Design review of the part built by this model. Coordinates are the model's own, in mm. Face numbers are marked on the shaded views. A direction names the side the tool comes from. Coordinates: 2 decimals unless noted, no trailing zeros. Loops run counter-clockwise (first coordinate to the right, second up) from the corner with the lowest first, then second, coordinate; pieces in that order, holes last. Notation, with made-up numbers: M 2,-10.75 L 13,-10.75 A22 ccw 13,26.25 Z; hole C 21.25,84.25 d11. An arc over 180 degrees is marked long. One line per item, written item: value.
```python
from build123d import *

# Parameters (mm, degrees)
SKETCH1_R                = 1.6
BOSS_EXTRUDE1_DEPTH      = 10
CUT_EXTRUDE1_DEPTH       = 51.495476
FILLET1_R                = 0.5
BOSS_EXTRUDE2_DEPTH      = 10
BOSS_EXTRUDE2_DEPTH_BACK = 20
SKETCH3_R                = 1.5
SKETCH4_W                = 10
SKETCH4_H                = 10
CUT_EXTRUDE3_DEPTH       = 54.383453
SKETCH5_W                = 8.66368
SKETCH5_H                = 10
CUT_EXTRUDE5_DEPTH       = 54.831153
FILLET3_R                = 0.5
FILLET4_R                = 1


with BuildPart() as part:
    # Sketch1 → Boss-Extrude1 (new body)
    with BuildSketch(Plane(origin=(0, 0, 0), x_dir=(1, 0, 0), z_dir=(0, 1, 0))):
        with BuildLine():
            Line((0, 0), (23.162951, -23.162951))
            ThreePointArc((23.162951, -23.162951), (23.813269, -26.432322), (21.041631, -28.284271))
            Line((21.041631, -28.284271), (0, -28.284271))
            Line((0, -28.284271), (0, -34.284271))
            Line((0, -34.284271), (30.698485, -34.284271))
            ThreePointArc((30.698485, -34.284271), (35.317882, -31.197688), (34.234019, -25.748737))
            Line((34.234019, -25.748737), (4.242641, 4.242641))
            Line((4.242641, 4.242641), (0, 0))
        make_face()
        with Locations(Location((31.905592, -29.784271, 0), (0, 0, 270))):
            Circle(SKETCH1_R, mode=Mode.SUBTRACT)
    extrude(amount=BOSS_EXTRUDE1_DEPTH)

    # Sketch2 → Cut-Extrude1 (cut, through all)
    with BuildSketch(Plane(origin=(0, 10, 0), x_dir=(1, 0, 0), z_dir=(0, 1, 0))):
        with BuildLine():
            Line((1.414214, -1.414214), (9.899495, -9.899495))
            ThreePointArc((9.899495, -9.899495), (7.071068, -4.242641), (1.414214, -1.414214))
        make_face()
        Polygon((0, -28.284271), (0, -34.284271), (25.79899, -34.284271), (19.79899, -28.284271), align=None)
    extrude(amount=-CUT_EXTRUDE1_DEPTH, mode=Mode.SUBTRACT)

    # Fillet1
    fillet1_edges = [part.edges().sort_by_distance(p)[0] for p in [
        (4.242641, 5, -4.242641),
        (0, 5, 0),
        (19.79899, 5, 28.284271),
        (25.79899, 5, 34.284271),
        (1.414214, 5, 1.414214),
        (9.899495, 5, 9.899495),
    ]]
    fillet(fillet1_edges, radius=FILLET1_R)

    # Sketch3 → Boss-Extrude2 (add, two sides: drawn at the far end of the back side and taken through both)
    with BuildSketch(Plane(origin=(0, 10, 0), x_dir=(1, 0, 0), z_dir=(0, 1, 0)).offset(-BOSS_EXTRUDE2_DEPTH_BACK)):
        with BuildLine():
            Line((20.652543, -29.137825), (25.652543, -34.137825))
            ThreePointArc((25.652543, -34.137825), (25.814755, -34.246211), (26.006097, -34.284271))
            Line((26.006097, -34.284271), (30.698485, -34.284271))
            ThreePointArc((30.698485, -34.284271), (35.317882, -31.197688), (34.234019, -25.748737))
            Line((34.234019, -25.748737), (31.062446, -22.577164))
            ThreePointArc((31.062446, -22.577164), (30.738022, -22.360392), (30.355339, -22.284271))
            Line((30.355339, -22.284271), (22.284271, -22.284271))
            Line((22.284271, -22.284271), (23.162951, -23.162951))
            ThreePointArc((23.162951, -23.162951), (23.813269, -26.432322), (21.041631, -28.284271))
            Line((21.041631, -28.284271), (21.006097, -28.284271))
            ThreePointArc((21.006097, -28.284271), (20.544157, -28.59293), (20.652543, -29.137825))
        make_face()
        with Locations(Location((31.905592, -29.784271, 0), (0, 0, 270))):
            Circle(SKETCH3_R, mode=Mode.SUBTRACT)
    extrude(amount=BOSS_EXTRUDE2_DEPTH + BOSS_EXTRUDE2_DEPTH_BACK)

    # Sketch4 → Cut-Extrude3 (cut, through all)
    with BuildSketch(Plane(origin=(0, 0, 0), x_dir=(0.7071067811865515, 0, 0.7071067811865437), z_dir=(-0.7071067811865437, 0, 0.7071067811865515))):
        with Locations((36.514719, 5)):
            Rectangle(SKETCH4_W, SKETCH4_H)
    extrude(amount=CUT_EXTRUDE3_DEPTH, mode=Mode.SUBTRACT)

    # Sketch5 → Cut-Extrude5 (cut, through all)
    with BuildSketch(Plane(origin=(-4.242641, 0, 4.242641), x_dir=(0.7071067811865476, 0, 0.7071067811865476), z_dir=(-0.7071067811865476, 0, 0.7071067811865476))):
        with Locations((45.846559, 5)):
            Rectangle(SKETCH5_W, SKETCH5_H)
    extrude(amount=-CUT_EXTRUDE5_DEPTH, mode=Mode.SUBTRACT)

    # Fillet3
    fillet3_edges = [part.edges().sort_by_distance(p)[0] for p in [
        (22.284271, -5, 22.284271),
        (22.284271, 15, 22.284271),
    ]]
    fillet(fillet3_edges, radius=FILLET3_R)

    # Fillet4
    fillet4_edges = [part.edges().sort_by_distance(p)[0] for p in [
        (29.355339, 5, 29.355339),
        (33.59798, 5, 25.112698),
    ]]
    fillet(fillet4_edges, radius=FILLET4_R)


solid = part.part
```
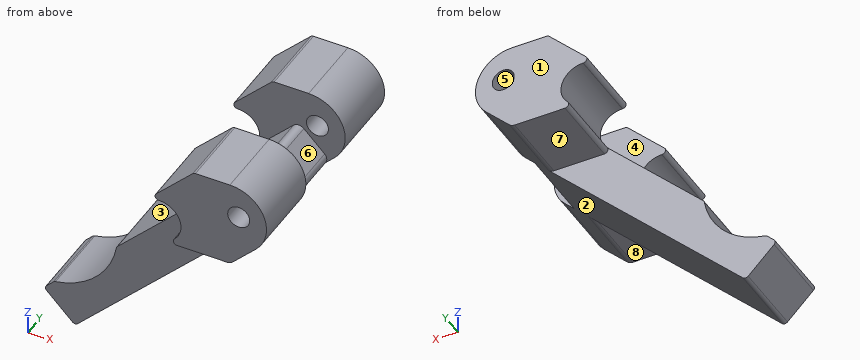
(1) Insertion check: pin 1 (6 mm diameter, centred on y = 10.5, z = 19, fed in from +X); pin 2 (2 mm diameter, centred on x = 27.5, y = 13, fed in from -Z); pin 3 (12 mm diameter, centred on x = 28.5, y = 6, fed in from -Z). Each pin has a flat end and moves straight along its axis. Give the tip position at first contact, or say it passes through.
Reply:
pin 1: stops at x = 30.44
pin 2: stops at z = 22.28
pin 3: stops at z = 14.01
(2) To check wall thickness, follow line 1 along Z through (x, y) = (31, 12.25); line 2 along Z through (x, y) = (29.5, -8.5); line 3 along Y through (x, z) = (27.5, 22). State the ranges of each line that lie inside material, in increasing order. Write a range as [from, to].
Reply:
line 1: z = [22.52, 28.59], [30.98, 34.28]
line 2: z = [22.28, 34.28]
line 3: y = [0, 10]
(3) Mouldability with a two-part tool opening along Y and no side actions: class the marked faces 1, 2 and 3 as released by +Y, released by -Y, zero draft, split by the parting line, or undercut.
Reply:
face 1: released by +Y
face 2: zero draft
face 3: undercut
(4) We need section B-B on x = 22.5. State the section outline as (y, z) points.
Reply:
outline: M -10,27.91 L 0,27.91 L 0,30.99 L -10,30.99 Z; M 0,14.01 L 10,14.01 L 10,22.5 L 0,22.5 Z; M 10,27.91 L 20,27.91 L 20,30.99 L 10,30.99 Z
(5) We need section D-D on y = 6. State the section outline as (x, z) points.
Reply:
outline: M 0.35,-0.35 L 3.89,-3.89 A0.5 ccw 4.6,-3.89 L 32.89,24.41 A1 ccw 32.89,25.82 L 30.06,28.65 A1 ccw 28.65,28.65 L 10.02,10.02 A0.5 ccw 9.88,9.74 A10 cw 1.57,1.44 A0.5 ccw 1.3,1.3 L 0.35,0.35 A0.5 ccw Z
(6) Tool access review of the marked faces 4, 5, 6, 7 and 8: name each direction out of +Z, -Z, +X, -X, +Y, -Y from which nothing blocks a thin tool from reaching the whole face with its end or side.
Reply:
face 4: +Z
face 5: +Y, -Y
face 6: +Z, +X
face 7: -Z, +X, -X, +Y
face 8: -Z, +X, -X, -Y
(7) We need section C-C on z = 30. State the section outline as (x, y) points.
Reply:
outline: M 21.51,-10 L 30.42,-10 L 30.42,0 L 21.51,0 Z; M 21.51,10 L 30.42,10 L 30.42,20 L 21.51,20 Z; M 33.39,-10 L 35.65,-10 L 35.65,0 L 33.39,0 Z; M 33.39,10 L 35.65,10 L 35.65,20 L 33.39,20 Z
